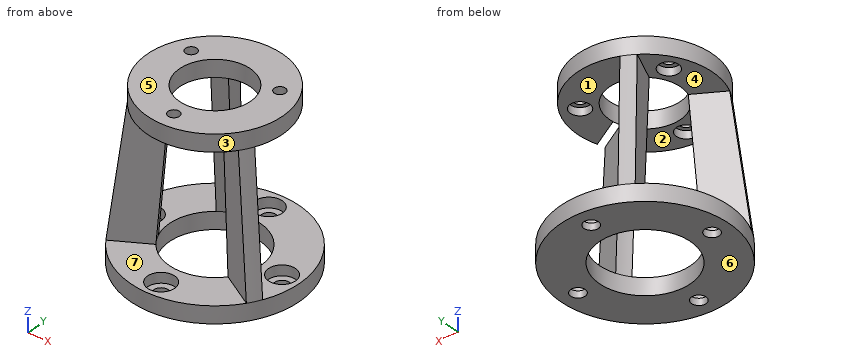
from build123d import *

# Parameters (mm, degrees)
F0_R     = 25
F0_R_2   = 2.15
F0_R_3   = 13.5
F1_DEPTH = 5
F2_R     = 4
F3_DEPTH = 3
F5_R     = 20
F5_R_2   = 1.65
F5_R_3   = 10.5
F6_DEPTH = 5
F7_R     = 2.9
F8_DEPTH = 2.3


with BuildPart() as f1:
    # F0 (on Top) → F1 (new body)
    with BuildSketch(Plane.XY):
        Circle(F0_R)
        with Locations((0, -19.65)):
            Circle(F0_R_2, mode=Mode.SUBTRACT)
        with Locations((-19.65, 0)):
            Circle(F0_R_2, mode=Mode.SUBTRACT)
        Circle(F0_R_3, mode=Mode.SUBTRACT)
        with Locations((19.65, 0)):
            Circle(F0_R_2, mode=Mode.SUBTRACT)
        with Locations((0, 19.65)):
            Circle(F0_R_2, mode=Mode.SUBTRACT)
    extrude(amount=F1_DEPTH)

    # F2 (on face) → F3 (cut)
    with BuildSketch(Plane.XY.offset(5)):
        with Locations((0, -19.65)):
            Circle(F2_R)
        with Locations((19.65, 0)):
            Circle(F2_R)
        with Locations((0, 19.65)):
            Circle(F2_R)
        with Locations((-19.65, 0)):
            Circle(F2_R)
    extrude(amount=-F3_DEPTH, mode=Mode.SUBTRACT)



with BuildPart() as f6:
    # F5 (on offset) → F6 (new body)
    with BuildSketch(Plane.XY.offset(44)):
        Circle(F5_R)
        with Locations((0, -15.011107)):
            Circle(F5_R_2, mode=Mode.SUBTRACT)
        with Locations((-13, 7.505553)):
            Circle(F5_R_2, mode=Mode.SUBTRACT)
        Circle(F5_R_3, mode=Mode.SUBTRACT)
        with Locations((13, 7.505553)):
            Circle(F5_R_2, mode=Mode.SUBTRACT)
    extrude(amount=F6_DEPTH)

    # F7 (on face) → F8 (cut)
    with BuildSketch(Plane(origin=(0, 0, 44), x_dir=(1, 0, 0), z_dir=(0, 0, -1))):
        with Locations((-13, -7.505553)):
            Circle(F7_R)
        with Locations((0, 15.011107)):
            Circle(F7_R)
        with Locations((13, -7.505553)):
            Circle(F7_R)
    extrude(amount=-F8_DEPTH, mode=Mode.SUBTRACT)


with BuildPart() as f1_1:
    add(f1.part)

    add(f6.part)  # F11 merges F6
    # F10 (on face) → F11 section 0
    with BuildSketch(Plane.XY.offset(5)):
        with BuildLine():
            ThreePointArc((12.562331, -4.943464), (11.691343, -6.75), (10.562331, -8.407566))
            Line((10.562331, -8.407566), (20.581242, -14.191987))
            ThreePointArc((20.581242, -14.191987), (21.650635, -12.5), (22.581242, -10.727885))
            Line((22.581242, -10.727885), (12.562331, -4.943464))
        make_face()
    # F9 (on face) → F11 section 1
    with BuildSketch(Plane(origin=(0, 0, 44), x_dir=(1, 0, 0), z_dir=(0, 0, -1))):
        with BuildLine():
            Line((9.926786, 3.421831), (18.233688, 8.217824))
            ThreePointArc((18.233688, 8.217824), (17.320508, 10), (16.233688, 11.681925))
            Line((16.233688, 11.681925), (7.926786, 6.885933))
            ThreePointArc((7.926786, 6.885933), (9.093267, 5.25), (9.926786, 3.421831))
        make_face()
    loft()

    # F9 (on face) → F12 section 0
    with BuildSketch(Plane(origin=(0, 0, 44), x_dir=(1, 0, 0), z_dir=(0, 0, -1))):
        with BuildLine():
            Line((-7.926786, 6.885933), (-16.233688, 11.681925))
            ThreePointArc((-16.233688, 11.681925), (-17.320508, 10), (-18.233688, 8.217824))
            Line((-18.233688, 8.217824), (-9.926786, 3.421831))
            ThreePointArc((-9.926786, 3.421831), (-9.093267, 5.25), (-7.926786, 6.885933))
        make_face()
    # F10 (on face) → F12 section 1
    with BuildSketch(Plane.XY.offset(5)):
        with BuildLine():
            ThreePointArc((-10.562331, -8.407566), (-11.691343, -6.75), (-12.562331, -4.943464))
            Line((-12.562331, -4.943464), (-22.581242, -10.727885))
            ThreePointArc((-22.581242, -10.727885), (-21.650635, -12.5), (-20.581242, -14.191987))
            Line((-20.581242, -14.191987), (-10.562331, -8.407566))
        make_face()
    loft()

    # F9 (on face) → F13 section 0
    with BuildSketch(Plane(origin=(0, 0, 44), x_dir=(1, 0, 0), z_dir=(0, 0, -1))):
        with BuildLine():
            Line((-7.287507, -7.559249), (-11.073882, -16.654403))
            ThreePointArc((-11.073882, -16.654403), (-9.345432, -17.682276), (-7.522499, -18.531379))
            Line((-7.522499, -18.531379), (-3.871069, -9.76037))
            ThreePointArc((-3.871069, -9.76037), (-5.686799, -8.826682), (-7.287507, -7.559249))
        make_face()
    # F10 (on face) → F13 section 1
    with BuildSketch(Plane.XY.offset(5)):
        with BuildLine():
            Line((-13.830633, 20.825792), (-8.221947, 10.707455))
            ThreePointArc((-8.221947, 10.707455), (-6.54493, 11.807366), (-4.723468, 12.646693))
            Line((-4.723468, 12.646693), (-10.332154, 22.76503))
            ThreePointArc((-10.332154, 22.76503), (-12.120241, 21.865493), (-13.830633, 20.825792))
        make_face()
    loft()


solid = f1_1.part
Verification items for the finished model (mm, model axes). Face numbers are marked on the shaded views. A direction names the side the tool comes from. Give positions to 0.01 mm unless a question says otherwise; leave off trailing zeros. Answer as CSV lines item,"result". Start each with the question number.
1. Sectioned sample at A-A (y = 0). Count the separate pieces of the cut face and the enclosed holes in it, then the cut area to 3 significant figures.
2. Set-up check for the marked faces 1, 2, 3 and 4: record each of +Z, -Z, +X, -X, +Y, -Y from which the full face is reachable in a straight line by a thin tool's end or side.
3. Thickness scan on line 1 (Y direction, x = 0, z = 1); line 2 (Y direction, x = 0, z = 48). Record the ranges inside material, lowest first.
4. Draft check along Z on the marked faces 5, 6 and 7. Enter one of: pulls with the +Z half, pulls with the -Z half, needs draft (parallel to the pull), parting line crosses it, or undercut.
5. Depth check by flat-ended pin: pin 1 (8 mm diameter, centred on y = -2.5, z = 34.5, fed in from -X); pin 2 (5 mm diameter, centred on y = 11, z = 28.5, fed in from -X); pin 3 (10 mm diameter, centred on y = -1.5, z = 37.5, fed in from +X); pin 4 (12.5 mm diameter, centred on x = 0, y = 0, fed in from +Z). Enter the tip coordinate at first touch or a pass-through.
Derived:
1,separate pieces,"6"
1,enclosed holes,"0"
1,area,"145 mm²"
2,face 1,"+X, +Y"
2,face 2,"-Y"
2,face 3,"+Z"
2,face 4,"-X"
3,line 1,"-25 to -21.8, -17.5 to -13.5, 13.5 to 17.5, 21.8 to 25"
3,line 2,"-20 to -16.66, -13.36 to -10.5, 10.5 to 20"
4,face 5,"pulls with the +Z half"
4,face 6,"pulls with the -Z half"
4,face 7,"undercut"
5,pin 1,"x = -15.26"
5,pin 2,"x = -9.89"
5,pin 3,"x = 15.26"
5,pin 4,"through"
